Input: part model. Units: mm. Frame: model coordinates. A direction names the side the tool comes from. Give positions to 0.01 mm unless a question says otherwise; leave off trailing zeros. Loops run counter-clockwise (first coordinate to the right, second up) from the corner with the lowest first, then second, coordinate; pieces in that order, holes last.
Autodesk Inventor part; units mm, degrees
ref_plane "YZ Plane" through (0, 0, 0) normal (1, 0, 0) x (0, 1, 0)
ref_plane "XZ Plane" through (0, 0, 0) normal (0, 1, 0) x (-1, 0, 0)
ref_plane "XY Plane" through (0, 0, 0) normal (0, 0, 1) x (1, 0, 0)
sketch "Sketch1" plane through (0, 0, 0) normal (1, 0, 0) x (0, 1, 0)
  line L0 (0, 0) -> (35, 0)
  line L1 (35, 0) -> (35, -86.8367)
  line L2 (35, -149) -> (0, -149)
  line L3 (0, -149) -> (0, 0)
  spline S0 degree 2 poles (35, -149) (46.832, -120.836) (35, -86.8367) knots 0 0 0 1 1 1
  point P0 (0, -76.4686)
  point P1 (40.9046, -120.7367)
  dimension "d0" = 35
  dimension "d1" = 149
extrude "Extrusion1" add sketch "Sketch1" against normal blind 6
properties part number "Inboard Wing Brace"
(1) Ray query, probe 1 along Y at (x, z) = (-0.25, -42.5); probe 2 along Y at (x, z) = (-1.5, -118.5). Return the intervals inside material, ascending.
Values follow:
probe 1: y = 0 to 35
probe 2: y = 0 to 40.91
(2) Cut plane A-A (z = -51). Return the cut outline in (x, y).
Values follow:
outline: (-6, 0) - (0, 0) - (0, 35) - (-6, 35) - close
(3) Reachability of faces 1 (the flat face through (-3, 0, -76)), 2 (the flat face through (-3, 35, -43)) from +Z, -Z, +X, -X, +Y, -Y: full face, straight path, thin tool, end or side. Return the list, or none.
Values follow:
face 1: +Z, -Z, +X, -X, -Y
face 2: +Z, +X, -X, +Y
(4) Pin query (flat end, axial travel): pin 1 Ø2 at (y, z) = (10, -47.5) entering from +X. Return the tip coordinate at first contact, or that it passes through.
Values follow:
pin 1: stops at x = 0
